Source: CAD feature listing. Evaluate the final solid. Frame: model axes, mm. A direction names the side the tool comes from. Round coordinates to 2 decimals unless told otherwise and drop trailing zeros. Loops run counter-clockwise (first coordinate to the right, second up) from the corner with the lowest first, then second, coordinate; pieces in that order, holes last. Notation, with made-up numbers: M 62.25,49.5 L 78.25,49.5 A18 cw 78.25,55.5 Z; hole C 69,-34.5 d7. An arc over 180 degrees is marked long. One line per item, written item: value.
from build123d import *

# Parameters (mm, degrees)
BOSS_EXTRUDE1_DEPTH  = 26
M4_CLEARANCE_HOLE1_D = 4.5
SKETCH5_R            = 7.5
CUT_EXTRUDE1_DEPTH   = 64.5
CHAMFER1_SIZE        = 6


with BuildPart() as part:
    # Sketch1 → Boss-Extrude1 (new body)
    with BuildSketch(Plane.XY):
        Polygon((0, 0), (0, 31.75), (3.175, 31.75), (3.175, 3.175), (63.5, 3.175), (63.5, 0), align=None)
    extrude(amount=BOSS_EXTRUDE1_DEPTH)

    # M4 Clearance Hole1 (through all)
    with Locations(Plane(origin=(0, 3.175, 0), x_dir=(1, 0, 0), z_dir=(0, 1, 0))):
        with Locations((23.175, -20.5), (23.175, -5.5), (48.175, -5.5), (48.175, -20.5)):
            Hole(M4_CLEARANCE_HOLE1_D / 2)

    # Sketch5 → Cut-Extrude1 (cut, through all)
    with BuildSketch(Plane.ZY):
        with Locations((13, 17.675)):
            Circle(SKETCH5_R)
    extrude(amount=-CUT_EXTRUDE1_DEPTH, mode=Mode.SUBTRACT)

    # Chamfer1
    chamfer1_edges = [part.edges().sort_by_distance(p)[0] for p in [
        (1.5875, 31.75, 26),
        (1.5875, 31.75, 0),
        (63.5, 1.5875, 0),
        (63.5, 1.5875, 26),
    ]]
    chamfer(chamfer1_edges, length=CHAMFER1_SIZE)


solid = part.part
1. Pull-direction query (X, two-part tool) for faces 3 (the face through (32, 0, 13)), 4 (the face through (23.663, 1.565, 22.696)), 5 (the face through (24.833, 1.565, 3.979)), 6 (the face through (3.175, 11, 19)); classes: released by +X, released by -X, zero draft, split by the parting line, or undercut.
Report:
face 3: zero draft
face 4: undercut
face 5: undercut
face 6: released by +X
2. Ray query, line 1 (Y direction, x = 1.35, z = 13) (3 decimals); line 2 (X direction, y = 2.2, z = 20.5) (3 decimals); line 3 (Y direction, x = 42, z = 17.25) (3 decimals). Return the intervals inside material, ascending. Write a range as [from, to].
Report:
line 1: y = [0, 10.175], [25.175, 31.75]
line 2: x = [0, 20.925], [25.425, 45.925], [50.425, 63]
line 3: y = [0, 3.175]
3. Section query D-D (z = 2.25). Return the cut outline in (x, y) (3 decimals), and give its area (3 significant figures).
Report:
outline: M 0,0 L 59.75,0 L 59.75,3.175 L 3.175,3.175 L 3.175,28 L 0,28 Z
area: 269 mm2
4. Section query B-B (z = 19). Return the cut outline in (x, y) (3 decimals).
Report:
outline: M 0,0 L 21.498,0 L 21.498,3.175 L 3.175,3.175 L 3.175,13.175 L 0,13.175 Z; M 0,22.175 L 3.175,22.175 L 3.175,31.75 L 0,31.75 Z; M 24.852,0 L 46.498,0 L 46.498,3.175 L 24.852,3.175 Z; M 49.852,0 L 63.5,0 L 63.5,3.175 L 49.852,3.175 Z
5. Reachability of faces 1 (the face through (33, 3.175, 13)), 2 (the face through (2, 31.75, 13)) from +Z, -Z, +X, -X, +Y, -Y: full face, straight path, thin tool, end or side. Return the list, or none.
Report:
face 1: +Z, -Z, +X, +Y
face 2: +Z, -Z, +X, -X, +Y
6. Section query C-C (y = 21.5). Return the cut outline in (x, z) (3 decimals), and give its area (3 significant figures).
Report:
outline: M 0,0 L 3.175,0 L 3.175,6.549 L 0,6.549 Z; M 0,19.451 L 3.175,19.451 L 3.175,26 L 0,26 Z
area: 41.6 mm2
7. Pin query (flat end, axial travel): pin 1 (8 mm diameter, centred on x = 49, z = 17.5, fed in from +Y) (3 decimals). Return the tip coordinate at first contact, or that it passes through.
Report:
pin 1: stops at y = 3.175
8. Section query A-A (z = 13). Return the cut outline in (x, y) (3 decimals).
Report:
outline: M 0,0 L 63.5,0 L 63.5,3.175 L 3.175,3.175 L 3.175,10.175 L 0,10.175 Z; M 0,25.175 L 3.175,25.175 L 3.175,31.75 L 0,31.75 Z
